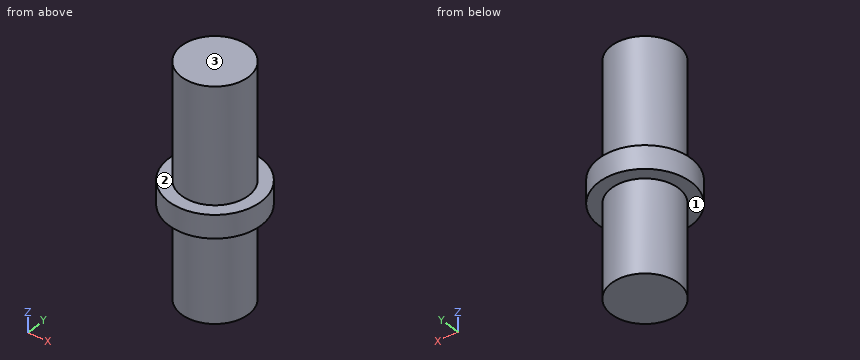
```python
from build123d import *

# Parameters (mm, degrees)
SKETCH2_R              = 2.9
LOCATOR_SHAFT_DEPTH    = 20
LOCATOR_SHOULDER_START = 8
SKETCH3_R              = 4
LOCATOR_SHOULDER_DEPTH = 2


with BuildPart() as part:
    # Sketch2 → Locator_shaft (new body)
    with BuildSketch(Plane.XY):
        Circle(SKETCH2_R)
    extrude(amount=LOCATOR_SHAFT_DEPTH)

    # Sketch3 → Locator_shoulder (add)
    with BuildSketch(Plane.XY.offset(LOCATOR_SHOULDER_START)):
        Circle(SKETCH3_R)
    extrude(amount=LOCATOR_SHOULDER_DEPTH)


solid = part.part
```
For this review, take the finished solid that the model builds, in its own axes (mm). Face numbers are marked on the shaded views. A direction names the side the tool comes from. Coordinates: 2 decimals unless noted, no trailing zeros. Write each loop counter-clockwise with the first axis right and the second up, starting at its lowest first coordinate (ties: lowest second). Pieces come first, ordered by that corner, then holes. Notation, with made-up numbers: (51.5, -28.75) -> (82.5, -28.75) arc R12 ccw to (82.5, -17.75) -> close; hole circle Ø4 at (17, 83.5). An arc over 180 degrees is marked (long way). Put each result on its own line as item: value.
Q1. Take a section at C-C, the plane z = 4.25. State the section outline as (x, y) points.
From the geometry:
outline: circle Ø5.8 at (0, 0)
Q2. Wall thickness on L1, parallel to Z at x = -0.5, y = 3.75; L2, parallel to Y at x = -0.5, z = 4.5; L3, parallel to Y at x = 3, z = 8.25: over which ranges is each line inside the solid? List them lowest first.
From the geometry:
L1: z = 8 to 10
L2: y = -2.86 to 2.86
L3: y = -2.65 to 2.65
Q3. Clearance check with flat-ended pins moving along their axes: pin 1 Ø2 at (y, z) = (-3, 9) entering from +X; pin 2 Ø1 at (y, z) = (-2, 6) entering from -X; pin 3 Ø1.5 at (y, z) = (1, 14) entering from -X. State where each tip first meets the part, or that it passes through.
From the geometry:
pin 1: stops at x = 3.46
pin 2: stops at x = -2.48
pin 3: stops at x = -2.89
Q4. Tool access review of the marked faces 1, 2 and 3: name each direction out of +Z, -Z, +X, -X, +Y, -Y from which nothing blocks a thin tool from reaching the whole face with its end or side.
From the geometry:
face 1: -Z
face 2: +Z
face 3: +Z, +X, -X, +Y, -Y
Q5. Take a section at A-A, the plane x = 0. State the section outline as (y, z) points.
From the geometry:
outline: (-4, 8) -> (-2.9, 8) -> (-2.9, 0) -> (2.9, 0) -> (2.9, 8) -> (4, 8) -> (4, 10) -> (2.9, 10) -> (2.9, 20) -> (-2.9, 20) -> (-2.9, 10) -> (-4, 10) -> close
